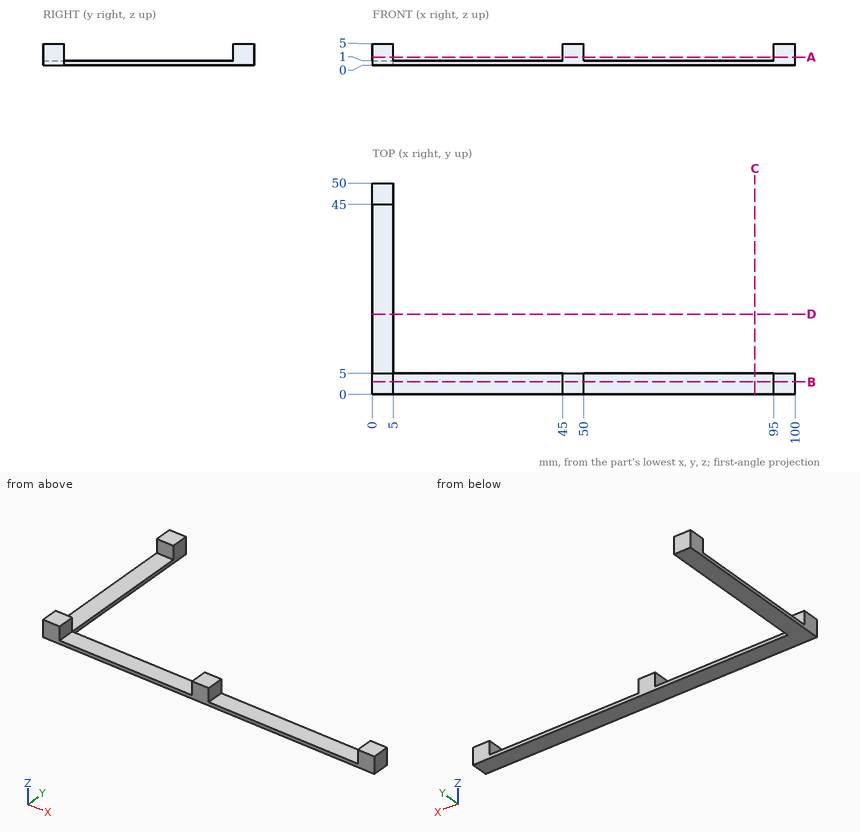
Job drawing, mm, ordinate dimensions from the low corner. One solid piece. Give positions to 0.01 mm unless a question says otherwise; leave off trailing zeros. Loops run counter-clockwise (first coordinate to the right, second up) from the corner with the lowest first, then second, coordinate; pieces in that order, holes last. Notation, with made-up numbers: (34.25, 30.5) -> (88.25, 30.5) arc R33 cw to (88.25, 65.5) -> close; hole circle Ø4 at (83, -19.5). An arc over 180 degrees is marked (long way). Use a Markdown table: item, result. Add a question column.
(1) Slice it at B-B on y = 3. List the corners of the cut face in (x, z).
(2) Wall check: line 1 along Z through (x, y) = (37.5, 2.5); line 2 along Y through (x, z) = (90.5, 0.3). Give the ranges that are in metal, low to high.
(3) Slice it at A-A on z = 1.9. List the corners of the cut face in (x, y).
(4) Drop flat-ended pins along their axis: pin 1 Ø2.5 at (y, z) = (16.5, 1.5) entering from +X; pin 2 Ø2.5 at (x, y) = (2, 17) entering from +Z; pin 3 Ø4 at (x, y) = (52, 8) entering from -Z; pin 4 Ø2 at (x, z) = (1.5, 3) entering from -Y. Give the stop position or say it passes through.
(5) Slice it at C-C on x = 90.5. List the corners of the cut face in (y, z).
Filled sheet:
| question | item | result |
|---|---|---|
| 1 | outline | (0, 0) -> (100, 0) -> (100, 5) -> (95, 5) -> (95, 1) -> (50, 1) -> (50, 5) -> (45, 5) -> (45, 1) -> (5, 1) -> (5, 5) -> (0, 5) -> close |
| 2 | line 1 | 0 to 1 |
| 2 | line 2 | 0 to 5 |
| 3 | outline | (0, 0) -> (5, 0) -> (5, 5) -> (0, 5) -> close; (0, 45) -> (5, 45) -> (5, 50) -> (0, 50) -> close; (45, 0) -> (50, 0) -> (50, 5) -> (45, 5) -> close; (95, 0) -> (100, 0) -> (100, 5) -> (95, 5) -> close |
| 4 | pin 1 | x = 5 |
| 4 | pin 2 | z = 1 |
| 4 | pin 3 | through |
| 4 | pin 4 | y = 0 |
| 5 | outline | (0, 0) -> (5, 0) -> (5, 1) -> (0, 1) -> close |
